Work out the finished part from the listing and answer in its coordinate system (mm). A direction names the side the tool comes from. Give positions to 0.01 mm unless a question says otherwise; leave off trailing zeros. Write each loop counter-clockwise with the first axis right and the second up, starting at its lowest first coordinate (ties: lowest second). Pieces come first, ordered by that corner, then holes. Notation, with made-up numbers: (63.5, 89.5) -> (84.5, 89.5) arc R33 cw to (84.5, 123.5) -> close; hole circle Ø6 at (12.25, 28). An arc over 180 degrees is marked (long way). Write item = value, one per line. Start each with the question number.
from build123d import *

# Parameters (mm, degrees)
F1_DEPTH = 3
F2_W     = 16
F2_H     = 1
F3_DEPTH = 10
F6_DEPTH = 10


with BuildPart() as f1:
    # F0 (on Top) → F1 (new body)
    with BuildSketch(Plane.XY):
        Polygon((0, -15), (0, 0), (-203, 0), (-203, 3), (-211, 3), (-225, 3), (-225, -17), (-216.947441, -47.052559), (-211, -53), (-211, -26), (-212, -26), (-212, -15), align=None)
        with BuildLine():
            Line((-211, 3), (-203, 3))
            ThreePointArc((-203, 3), (-205.111456, 11.944272), (-211, 19))
            Line((-211, 19), (-211, 3))
        make_face()
    extrude(amount=F1_DEPTH)

    # F2 (on face) → F3 (cut)
    with BuildSketch(Plane(origin=(-211, 0, 0), x_dir=(0, -1, 0), z_dir=(-1, 0, 0))):
        with Locations((-11, 2.5)):
            Rectangle(F2_W, F2_H)
    extrude(amount=-F3_DEPTH, mode=Mode.SUBTRACT)

    # F5 (on offset) → F6 (cut)
    with BuildSketch(Plane.XZ.offset(53)):
        Polygon((-214, 3), (-211, 1.5), (-214, 0), (-206, 0), (-206, 3), align=None)
    extrude(amount=-F6_DEPTH, mode=Mode.SUBTRACT)


solid = f1.part
(1) A cutting plane is placed at A-A, the plane z = 0.6. Write down the section's boundary in (x, y).
(2) Each of these flat-tipped pins is pushed along its axis until it touches: pin 1 (0.5 mm diameter, centred on x = -211.5, z = 2, fed in from +Y); pin 2 (4 mm diameter, centred on x = -209, y = 9.5, fed in from +Z); pin 3 (1 mm diameter, centred on x = -158, z = 2, fed in from +Y). Where does it stop, or does it pass through?
(3) Find the intervals of material crossed by line 1 along Y through (x, z) = (-194.5, 0.75); line 2 along X through (y, z) = (-23.5, 1.5); line 3 along X through (y, z) = (-27, 0.6), in increasing order.
(4) A cutting plane is placed at B-B, the plane x = -76.5. Write down the section's boundary in (y, z), then the cut area to 3 significant figures.
(5) For faces 1 (the flat face through (-130, -12, 3)), 2 (the flat face through (-208, 9, 2)), determine the directions among +Z, -Z, +X, -X, +Y, -Y from which every point of the face is accessible in a straight line to the end or side of a thin tool.
(6) A cutting plane is placed at C-C, the plane y = 11. Write down the section's boundary in (x, z).
Results list:
q1.outline = (-225, -17) -> (-216.95, -47.05) -> (-212.8, -51.2) -> (-212.8, -43) -> (-211, -43) -> (-211, -26) -> (-212, -26) -> (-212, -15) -> (0, -15) -> (0, 0) -> (-203, 0) -> (-203, 3) arc R20 ccw to (-211, 19) -> (-211, 3) -> (-225, 3) -> close
q2.pin_1 = 3
q2.pin_2 = 2
q2.pin_3 = 0
q3.line_1 = -15 to 0
q3.line_2 = -223.26 to -212
q3.line_3 = -222.32 to -211
q4.outline = (-15, 0) -> (0, 0) -> (0, 3) -> (-15, 3) -> close
q4.area = 45.0 mm²
q5.face_1 = +Z, +X, -X, +Y, -Y
q5.face_2 = +Z, +X, -X, +Y
q6.outline = (-211, 0) -> (-204.67, 0) -> (-204.67, 2) -> (-211, 2) -> close
